```python
from build123d import *

# Parameters (mm, degrees)
CROQUIS1_W              = 11.672108333
CROQUIS1_H              = 15.427149297
SALIENTE_EXTRUIR1_DEPTH = 60
CROQUIS2_R              = 4
CORTAR_EXTRUIR1_DEPTH   = 60
CROQUIS5_W              = 60
CROQUIS5_H              = 14.732368319
SALIENTE_EXTRUIR4_DEPTH = 5
CROQUIS6_W              = 14.792406449
CROQUIS6_H              = 16
CORTAR_EXTRUIR2_DEPTH   = 0.2
CORTAR_EXTRUIR3_DEPTH   = 60
SALIENTE_EXTRUIR5_DEPTH = 60


with BuildPart() as part:
    # Croquis1 → Saliente-Extruir1 (new body)
    with BuildSketch(Plane(origin=(0, 0, 0), x_dir=(0, 0, -1), z_dir=(1, 0, 0))):
        Polygon((0, 23.023275897), (6.259402679, 26.20509842), (15, 26.20509842), (16.468373545, 24.736724875), (30, 24.736724875), (36.2, 24.736724875), (36.2, 20.972943127), (30, 20.972943127), (30, 4.65930459), (36.2, 4.65930459), (36.2, 1.468373545), (30, 1.468373545), (16.468373545, 1.468373545), (15, 0), (6.259402679, 0), (0, 3.181822522), (0, 5.10254921), (15, 5.10254921), (15, 21.10254921), (0, 21.10254921), align=None)
        with Locations((22.807201834, 12.816123859)):
            Rectangle(CROQUIS1_W, CROQUIS1_H, mode=Mode.SUBTRACT)
    extrude(amount=SALIENTE_EXTRUIR1_DEPTH)

    # Croquis2 → Cortar-Extruir1 (cut)
    with BuildSketch(Plane(origin=(0, 24.736724875, 0), x_dir=(1, 0, 0), z_dir=(0, 1, 0))):
        with Locations(Location((30, 22.555814773, 0), (0, 0, 270))):
            Circle(CROQUIS2_R)
    extrude(amount=-CORTAR_EXTRUIR1_DEPTH, mode=Mode.SUBTRACT)

    # Croquis5 → Saliente-Extruir4 (add)
    with BuildSketch(Plane(origin=(0, 5.10254921, 0), x_dir=(1, 0, 0), z_dir=(0, 1, 0))):
        with Locations((30, 7.633815841)):
            Rectangle(CROQUIS5_W, CROQUIS5_H)
    saliente_extruir4 = extrude(amount=SALIENTE_EXTRUIR4_DEPTH)

    # Simetría1: Saliente-Extruir4 across plane
    add(saliente_extruir4.mirror(Plane.ZX.offset(13.10254921)))

    # Croquis6 → Cortar-Extruir2 (cut)
    with BuildSketch(Plane(origin=(60, 0, 0), x_dir=(0, 0, -1), z_dir=(1, 0, 0))):
        with Locations((7.663834905, 13.10254921)):
            Rectangle(CROQUIS6_W, CROQUIS6_H)
    cortar_extruir2 = extrude(amount=-CORTAR_EXTRUIR2_DEPTH, mode=Mode.SUBTRACT)

    # Simetría2: Cortar-Extruir2 across plane
    add(cortar_extruir2.mirror(Plane(origin=(30, 0, 0), x_dir=(0, 0, 1), z_dir=(1, 0, 0))), mode=Mode.SUBTRACT)

    # Croquis7 → Cortar-Extruir3 (cut)
    with BuildSketch(Plane(origin=(60, 0, 0), x_dir=(0, 0, -1), z_dir=(1, 0, 0))):
        Polygon((16.040272261, 1.040272261), (4.212939392, 1.040272261), (2.720078376, -1.896540894), (18.763264408, -1.896540894), align=None)
    extrude(amount=-CORTAR_EXTRUIR3_DEPTH, mode=Mode.SUBTRACT)

    # Croquis8 → Saliente-Extruir5 (add)
    with BuildSketch(Plane.ZY):
        Polygon((-27.827964964, 1.040272261), (-36.2, 1.040272261), (-36.2, 1.468373545), (-27.399863681, 1.468373545), align=None)
    extrude(amount=-SALIENTE_EXTRUIR5_DEPTH)


solid = part.part
```
CAD build for the part. Positions are in the model's coordinates, mm. A direction names the side the tool comes from. Coordinates: 2 decimals unless noted, no trailing zeros. Loops run counter-clockwise (first coordinate to the right, second up) from the corner with the lowest first, then second, coordinate; pieces in that order, holes last. Notation, with made-up numbers: (-34.75, -25) - (22.25, -25) arc R10 cw to (22.25, -16) - close; hole circle Ø3 at (-36, 37). An arc over 180 degrees is marked (long way). Use CSV: the item, a comma, the result in double quotes. Start each with the question number.
Q1. Probe probe 1 along Y at (x, z) = (37, -23.5); probe 2 along Z at (x, y) = (53.5, 16.25); probe 3 along Z at (x, y) = (47, 15.75). List the from-to ranges inside material, lowest first. Write a range as from..to.
Q2. Cut at D-D, the plane z = -24. List the corners of the cut face in (x, y), then the cut area to 3 significant figures.
Q3. Cut at B-B, the plane x = 20. List the corners of the cut face in (y, z).
Q4. Drop flat-ended pins along their axis: P1, Ø10, axis at x = 36, z = -26.5, coming from the +Y side; P2, Ø4, axis at x = 29.5, y = 18.5, coming from the +Z side; P3, Ø12, axis at x = 32.5, y = 13.5, coming from the -Z side. Give the stop position or say it passes through.
Q5. Cut at C-C, the plane y = 17.5. List the corners of the cut face in (x, z), then the cut area to 3 significant figures.
Q6. Two-plate mould, pull along X, no slides. Class faces 4 (the cylindrical face through (31.2, 3.31, -18.74)), 5 (the flat face through (0.2, 9.7, -7.6)), 6 (the flat face through (30, 13, -28.643)): +X half, -X half, draft (parallel to the pull), parting line (faces both ways), or undercut.
Q7. Cut at A-A, the plane z = -8. List the corners of the cut face in (x, y).
Q8. 3-axis set-ups, long thin cutter, end or side, ignore diameter. For faces 1 (the flat face through (30, 5.103, -27)), 2 (the flat face through (30, 8, -0.268)), 3 (the flat face through (30, 4.659, -33)): which of +Z, -Z, +X, -X, +Y, -Y reach the whole face in a straight line?
Here are the results:
1,probe 1,"1.47..5.1, 20.53..24.74"
1,probe 2,"-30..-28.64, -16.97..-0.27"
1,probe 3,"-30..-28.64, -16.97..-15"
2,outline,"(0, 1.47) - (26.27, 1.47) - (26.27, 5.1) - (0, 5.1) - close; (0, 20.53) - (26.27, 20.53) - (26.27, 24.74) - (0, 24.74) - close; (33.73, 1.47) - (60, 1.47) - (60, 5.1) - (33.73, 5.1) - close; (33.73, 20.53) - (60, 20.53) - (60, 24.74) - (33.73, 24.74) - close"
2,area,"412 mm2"
3,outline,"(1.04, -36.2) - (4.66, -36.2) - (4.66, -30) - (20.97, -30) - (20.97, -36.2) - (24.74, -36.2) - (24.74, -16.47) - (26.21, -15) - (26.21, -6.26) - (23.02, 0) - (21.1, 0) - (21.1, -0.27) - (16.1, -0.27) - (16.1, -15) - (10.1, -15) - (10.1, -0.27) - (5.1, -0.27) - (5.1, 0) - (3.18, 0) - (1.04, -4.21) - (1.04, -16.04) - (1.47, -16.47) - (1.47, -27.4) - (1.04, -27.83) - close; hole (5.1, -28.64) - (20.53, -28.64) - (20.53, -16.97) - (5.1, -16.97) - close"
4,P1,"y = 24.74"
4,P2,"z = -0.27"
4,P3,"z = -30"
5,outline,"(0, -30) - (60, -30) - (60, -28.64) - (0, -28.64) - close; (0, -16.97) - (60, -16.97) - (60, -15.06) - (59.8, -15.06) - (59.8, -0.27) - (0.2, -0.27) - (0.2, -15.06) - (0, -15.06) - close"
5,area,"1,080 mm2"
6,face 4,"undercut"
6,face 5,"-X half"
6,face 6,"draft"
7,outline,"(0, 1.04) - (60, 1.04) - (60, 5.1) - (59.8, 5.1) - (59.8, 10.1) - (0.2, 10.1) - (0.2, 5.1) - (0, 5.1) - close; (0, 21.1) - (0.2, 21.1) - (0.2, 16.1) - (59.8, 16.1) - (59.8, 21.1) - (60, 21.1) - (60, 26.21) - (0, 26.21) - close"
8,face 1,"+X, -X"
8,face 2,"+Z, +X, -X"
8,face 3,"-Z, +X, -X"
